from build123d import *

# Parameters (mm, degrees)
F1_DEPTH = 12.7
F2_R     = 0.3


# Not quite as in the source:
# - a feature names something its author has since deleted; it is built from what else it names


with BuildPart() as f1:
    # F0 (on Front) → F1 (new body, symmetric)
    with BuildSketch(Plane.XZ):
        Polygon((0, 25.4), (0, 0), (2.5, 0), (2.5, 3), (11.1, 3), (11.1, 0), (13.6, 0), (13.6, 25.4), (10.855, 25.4), (10.855, 22.4), (2.745, 22.4), (2.745, 25.4), align=None)
    extrude(amount=F1_DEPTH, both=True)

    # F2
    f2_edges = [f1.edges().sort_by_distance(p)[0] for p in [
        (0, 12.7, 12.7),
        (0, -12.7, 12.7),
        (0, 0, 0),
        (1.25, -12.7, 0),
        (13.6, -12.7, 12.7),
        (13.6, 12.7, 12.7),
        (1.25, 12.7, 0),
        (6.8, -12.7, 22.4),
        (2.745, -12.7, 23.9),
        (2.745, 0, 25.4),
        (10.855, -12.7, 23.9),
        (10.855, 0, 25.4),
        (2.745, 0, 22.4),
        (6.8, 12.7, 22.4),
        (10.855, 0, 22.4),
        (2.5, 0, 3),
        (2.5, -12.7, 1.5),
        (6.8, -12.7, 3),
        (11.1, -12.7, 1.5),
        (11.1, 0, 0),
        (12.35, -12.7, 0),
        (2.5, 12.7, 1.5),
        (6.8, 12.7, 3),
        (11.1, 12.7, 1.5),
        (11.1, 0, 3),
        (12.2275, -12.7, 25.4),
        (1.3725, -12.7, 25.4),
        (1.3725, 12.7, 25.4),
        (12.2275, 12.7, 25.4),
        (12.35, 12.7, 0),
        (0, 0, 25.4),
        (2.745, 12.7, 23.9),
        (10.855, 12.7, 23.9),
        (13.6, 0, 25.4),
        (13.6, 0, 0),
        (2.5, 0, 0),
    ]]
    fillet(f2_edges, radius=F2_R)


solid = f1.part
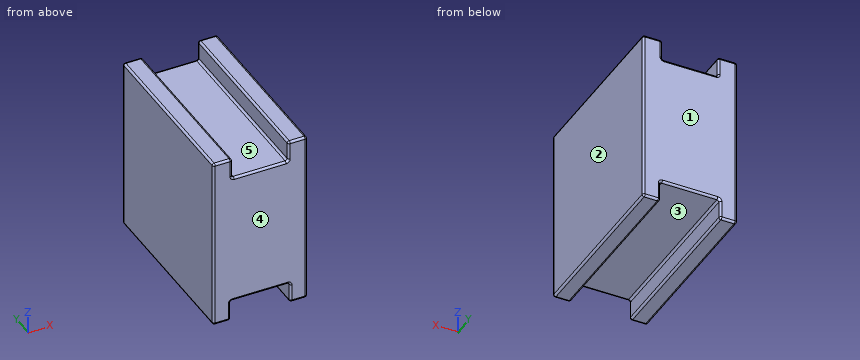
Source: CAD feature listing. Evaluate the final solid. Frame: model axes, mm. Face numbers are marked on the shaded views. A direction names the side the tool comes from. Round coordinates to 2 decimals unless told otherwise and drop trailing zeros. Loops run counter-clockwise (first coordinate to the right, second up) from the corner with the lowest first, then second, coordinate; pieces in that order, holes last.
Q1. Section A-A, the plane x = 5. Return loops of the section in (y, z), plus the area to 3 significant figures.
Q2. Mould query, pull axis X, two halves, no side actions, for the marked faces 1, 2 and 3. Classes: pulls with the +X half, pulls with the -X half, needs draft (parallel to the pull), parting line crosses it, or undercut.
Q3. Ray query, line 1 (X direction, y = 4.5, z = 22.75) (3 decimals); line 2 (Z direction, x = 5.5, y = 3.75); line 3 (Z direction, x = 11.25, y = -3.25). Return the intervals inside material, ascending.
Q4. First-contact query: P1, Ø1.5, axis at x = 5.5, y = 2, coming from the +Z side; P2, Ø3, axis at x = 3, y = 3.5, coming from the +Z side. Flat tips, straight axial feed; report the tip coordinate or a pass-through.
Q5. Section B-B, the plane y = -8.5. Return loops of the section in (x, z) (3 decimals), plus the area to 3 significant figures.
Q6. Access query for the marked faces 4 and 5. Directions: +Z, -Z, +X, -X, +Y, -Y. A direction counts if a zero-diameter tool reaches every point of the face in a straight line with its end or side. Return the directions, or none.
Solutions:
1. outline: (-12.7, 3.3) arc R0.3 ccw to (-12.4, 3) - (12.4, 3) arc R0.3 ccw to (12.7, 3.3) - (12.7, 22.1) arc R0.3 ccw to (12.4, 22.4) - (-12.4, 22.4) arc R0.3 ccw to (-12.7, 22.1) - close
1. area: 493 mm2
2. face 1: needs draft
2. face 2: pulls with the +X half
2. face 3: undercut
3. line 1: x = 0 to 2.745, 10.855 to 13.6
3. line 2: z = 3 to 22.4
3. line 3: z = 0.04 to 25.4
4. P1: stops at z = 22.4
4. P2: stops at z = 25.4
5. outline: (0, 0.3) arc R0.3 ccw to (0.3, 0) - (2.2, 0) arc R0.3 ccw to (2.5, 0.3) - (2.5, 2.7) arc R0.3 cw to (2.8, 3) - (10.8, 3) arc R0.3 cw to (11.1, 2.7) - (11.1, 0.3) arc R0.3 ccw to (11.4, 0) - (13.3, 0) arc R0.3 ccw to (13.6, 0.3) - (13.6, 25.1) arc R0.3 ccw to (13.3, 25.4) - (11.155, 25.4) arc R0.3 ccw to (10.855, 25.1) - (10.855, 22.7) arc R0.3 cw to (10.555, 22.4) - (3.045, 22.4) arc R0.3 cw to (2.745, 22.7) - (2.745, 25.1) arc R0.3 ccw to (2.445, 25.4) - (0.3, 25.4) arc R0.3 ccw to (0, 25.1) - close
5. area: 295 mm2
6. face 4: +Z, -Z, +X, -X, -Y
6. face 5: +Z, +Y, -Y
